For this review, take the finished solid that the model builds, in its own axes (mm). Face numbers are marked on the shaded views. A direction names the side the tool comes from. Give positions to 0.01 mm unless a question says otherwise; leave off trailing zeros. Loops run counter-clockwise (first coordinate to the right, second up) from the corner with the lowest first, then second, coordinate; pieces in that order, holes last. Notation, with made-up numbers: (14.5, -39) - (24.5, -39) arc R17 cw to (24.5, -33) - close; hole circle Ø2 at (69.5, 72.25). An arc over 180 degrees is marked (long way). Put each result on its own line as item: value. Start each with the question number.
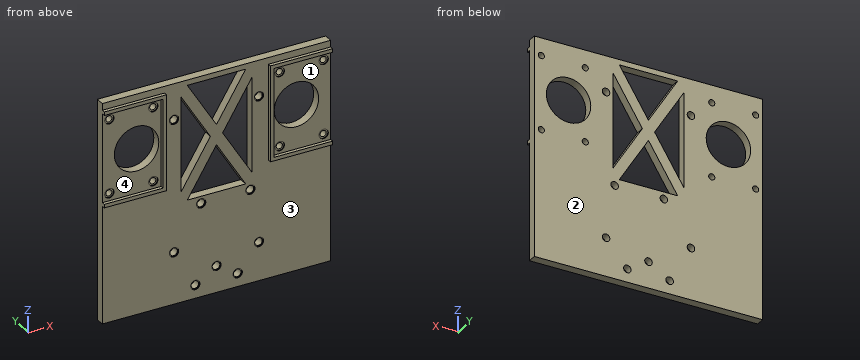
from build123d import *

# Parameters (mm, degrees)
SKETCH1_W           = 130
SKETCH1_H           = 125
BOSS_EXTRUDE1_DEPTH = 5
SKETCH2_R           = 1.75
SKETCH2_R_2         = 12.65
CUT_EXTRUDE1_DEPTH  = 10
SKETCH3_R           = 2.15
CUT_EXTRUDE2_DEPTH  = 10
SKETCH4_R           = 2.15
CUT_EXTRUDE3_DEPTH  = 10
BOSS_EXTRUDE2_DEPTH = 2
SKETCH6_R           = 2.65
CUT_EXTRUDE4_DEPTH  = 0.5
CUT_EXTRUDE5_DEPTH  = 91.311959341


with BuildPart() as part:
    # Sketch1 → Boss-Extrude1 (new body)
    with BuildSketch(Plane(origin=(0, 0, 0), x_dir=(1, 0, 0), z_dir=(0, 1, 0))):
        Rectangle(SKETCH1_W, SKETCH1_H)
    extrude(amount=BOSS_EXTRUDE1_DEPTH)

    # Sketch2 → Cut-Extrude1 (cut)
    with BuildSketch(Plane(origin=(0, 5, 0), x_dir=(1, 0, 0), z_dir=(0, 1, 0))):
        with Locations(Location((-61, -52.5, 0), (0, 0, 270))):
            Circle(SKETCH2_R)
        with Locations(Location((-36, -52.5, 0), (0, 0, 270))):
            Circle(SKETCH2_R)
        with Locations(Location((-36, -10.5, 0), (0, 0, 270))):
            Circle(SKETCH2_R)
        with Locations(Location((-61, -10.5, 0), (0, 0, 270))):
            Circle(SKETCH2_R)
        with Locations(Location((-45.5, -31.5, 0), (0, 0, 270))):
            Circle(SKETCH2_R_2)
    cut_extrude1 = extrude(amount=-CUT_EXTRUDE1_DEPTH, mode=Mode.SUBTRACT)

    # Mirror3: Cut-Extrude1 across plane
    add(cut_extrude1.mirror(Plane.ZY), mode=Mode.SUBTRACT)

    # Sketch3 → Cut-Extrude2 (cut)
    with BuildSketch(Plane(origin=(0, 5, 0), x_dir=(1, 0, 0), z_dir=(0, 1, 0))):
        with Locations(Location((-24.17, -42.03, 0), (0, 0, 270))):
            Circle(SKETCH3_R)
        with Locations(Location((24.17, -42.03, 0), (0, 0, 270))):
            Circle(SKETCH3_R)
        with Locations(Location((-8.73, 9.6, 0), (0, 0, 270))):
            Circle(SKETCH3_R)
        with Locations(Location((19.29, 9.6, 0), (0, 0, 270))):
            Circle(SKETCH3_R)
        with Locations(Location((-24.17, 33.11, 0), (0, 0, 270))):
            Circle(SKETCH3_R)
        with Locations(Location((24.17, 40.6, 0), (0, 0, 270))):
            Circle(SKETCH3_R)
    extrude(amount=-CUT_EXTRUDE2_DEPTH, mode=Mode.SUBTRACT)

    # Sketch4 → Cut-Extrude3 (cut)
    with BuildSketch(Plane(origin=(0, 5, 0), x_dir=(1, 0, 0), z_dir=(0, 1, 0))):
        with Locations(Location((0, 47.5, 0), (0, 0, 270))):
            Circle(SKETCH4_R)
        with Locations(Location((12.049810205, 55, 0), (0, 0, 270))):
            Circle(SKETCH4_R)
        with Locations(Location((-12.049810205, 55, 0), (0, 0, 270))):
            Circle(SKETCH4_R)
    extrude(amount=-CUT_EXTRUDE3_DEPTH, mode=Mode.SUBTRACT)

    # Sketch5 → Boss-Extrude2 (add)
    with BuildSketch(Plane.XZ):
        Polygon((-65, 58.7), (-65, 56.7), (-31.6, 56.7), (-31.6, 6.3), (-65, 6.3), (-65, 4.3), (-29.6, 4.3), (-29.6, 58.7), align=None)
    boss_extrude2 = extrude(amount=BOSS_EXTRUDE2_DEPTH)

    # Mirror5: Boss-Extrude2 across plane
    add(boss_extrude2.mirror(Plane.ZY))

    # Sketch6 → Cut-Extrude4 (cut)
    with BuildSketch(Plane.XZ):
        with Locations(Location((-12.049810205, -55, 0), (0, 0, 270))):
            Circle(SKETCH6_R)
        with Locations(Location((12.049810205, -55, 0), (0, 0, 270))):
            Circle(SKETCH6_R)
        with Locations(Location((0, -47.5, 0), (0, 0, 270))):
            Circle(SKETCH6_R)
        with Locations(Location((24.17, -40.6, 0), (0, 0, 270))):
            Circle(SKETCH6_R)
        with Locations(Location((-24.17, -33.11, 0), (0, 0, 270))):
            Circle(SKETCH6_R)
        with Locations(Location((-8.73, -9.6, 0), (0, 0, 270))):
            Circle(SKETCH6_R)
        with Locations(Location((19.29, -9.6, 0), (0, 0, 270))):
            Circle(SKETCH6_R)
        with Locations(Location((-61, 10.5, 0), (0, 0, 270))):
            Circle(SKETCH6_R)
        with Locations(Location((-61, 52.5, 0), (0, 0, 270))):
            Circle(SKETCH6_R)
        with Locations(Location((-36, 52.5, 0), (0, 0, 270))):
            Circle(SKETCH6_R)
        with Locations(Location((-36, 10.5, 0), (0, 0, 270))):
            Circle(SKETCH6_R)
        with Locations(Location((-24.17, 42.03, 0), (0, 0, 270))):
            Circle(SKETCH6_R)
        with Locations(Location((24.17, 42.03, 0), (0, 0, 270))):
            Circle(SKETCH6_R)
        with Locations(Location((36, 52.5, 0), (0, 0, 270))):
            Circle(SKETCH6_R)
        with Locations(Location((36, 10.5, 0), (0, 0, 270))):
            Circle(SKETCH6_R)
        with Locations(Location((61, 10.5, 0), (0, 0, 270))):
            Circle(SKETCH6_R)
        with Locations(Location((61, 52.5, 0), (0, 0, 270))):
            Circle(SKETCH6_R)
    extrude(amount=-CUT_EXTRUDE4_DEPTH, mode=Mode.SUBTRACT)

    # Sketch7 → Cut-Extrude5 (cut, through all)
    with BuildSketch(Plane.XZ):
        Polygon((-3.470107527, 26.95), (-20.17, 53.9), (-20.17, 0), align=None)
        Polygon((16.629937096, 59.5), (-16.629937096, 59.5), (0, 32.662892788), align=None)
        Polygon((20.17, 0), (20.17, 53.9), (3.470107527, 26.95), align=None)
        Polygon((0, 21.237107212), (-16.629937096, -5.6), (16.629937096, -5.6), align=None)
    extrude(amount=-CUT_EXTRUDE5_DEPTH, mode=Mode.SUBTRACT)


solid = part.part
1) Insertion check: P1, Ø16.5, axis at x = 43.5, z = 37.5, coming from the -Y side; P2, Ø4.5, axis at x = 36, z = 52.5, coming from the -Y side; P3, Ø3, axis at x = 36, z = 10.5, coming from the +Y side; P4, Ø2, axis at y = -1.5, z = 29.5, coming from the -X side. Each pin has a flat end and moves straight along its axis. Give the tip position at first contact, or say it passes through.
2) Take a section at C-C on x = 45.5. State the section outline as (y, z) points, and give its area (4 significant figures).
3) Take a section at B-B on z = -47.5. State the section outline as (x, y) points.
4) Mouldability with a two-part tool opening along Z and no side actions: class the marked faces 3 and 4 as released by +Z, released by -Z, zero draft, split by the parting line, or undercut.
5) Machinability: for the marked faces 1 and 2, which of the approach directions +Z, -Z, +X, -X, +Y, -Y give a long, thin tool a straight path to every point of the face, cutting with its end or side? Answer none if there is none.
6) Take a section at D-D on x = -36. State how many separate pieces and enclosed holes the cut face has, and give its area (3 significant figures).
7) Take a section at A-A on x = 24.17. State the section outline as (y, z) points.
8) Wall thickness on probe 1 along X at (y, z) = (0.3, -55); probe 2 along Z at (x, y) = (20, 4.5); probe 3 along Z at (x, y) = (5, 0.75): over which ranges is each line inside the solid? List them lowest first.
Answers follow:
1. P1: y = 0
1. P2: y = 0.5
1. P3: through
1. P4: x = -31.6
2. outline: (-2, 4.3) - (0, 4.3) - (0, -62.5) - (5, -62.5) - (5, 18.85) - (0, 18.85) - (0, 6.3) - (-2, 6.3) - close; (-2, 56.7) - (0, 56.7) - (0, 44.15) - (5, 44.15) - (5, 62.5) - (0, 62.5) - (0, 58.7) - (-2, 58.7) - close
2. area: 506.5 mm2
3. outline: (-65, 0) - (-2.65, 0) - (-2.65, 0.5) - (-2.15, 0.5) - (-2.15, 5) - (-65, 5) - close; (2.15, 0.5) - (2.65, 0.5) - (2.65, 0) - (65, 0) - (65, 5) - (2.15, 5) - close
4. face 3: zero draft
4. face 4: undercut
5. face 1: +X, -Y
5. face 2: +Z, -Z, +X, -X, +Y
6. separate pieces: 4
6. enclosed holes: 0
6. area: 513 mm2
7. outline: (0, -62.5) - (5, -62.5) - (5, -42.75) - (0.5, -42.75) - (0.5, -43.25) - (0, -43.25) - close; (0, -37.95) - (0.5, -37.95) - (0.5, -38.45) - (5, -38.45) - (5, 39.88) - (0.5, 39.88) - (0.5, 39.38) - (0, 39.38) - close; (0, 44.68) - (0.5, 44.68) - (0.5, 44.18) - (5, 44.18) - (5, 62.5) - (0, 62.5) - close
8. probe 1: -65 to -14.7, -9.4 to 9.4, 14.7 to 65
8. probe 2: -62.5 to -11.63, -7.57 to 0.27, 53.63 to 62.5
8. probe 3: -62.5 to -5.6, 13.17 to 24.48, 29.42 to 40.73, 59.5 to 62.5
